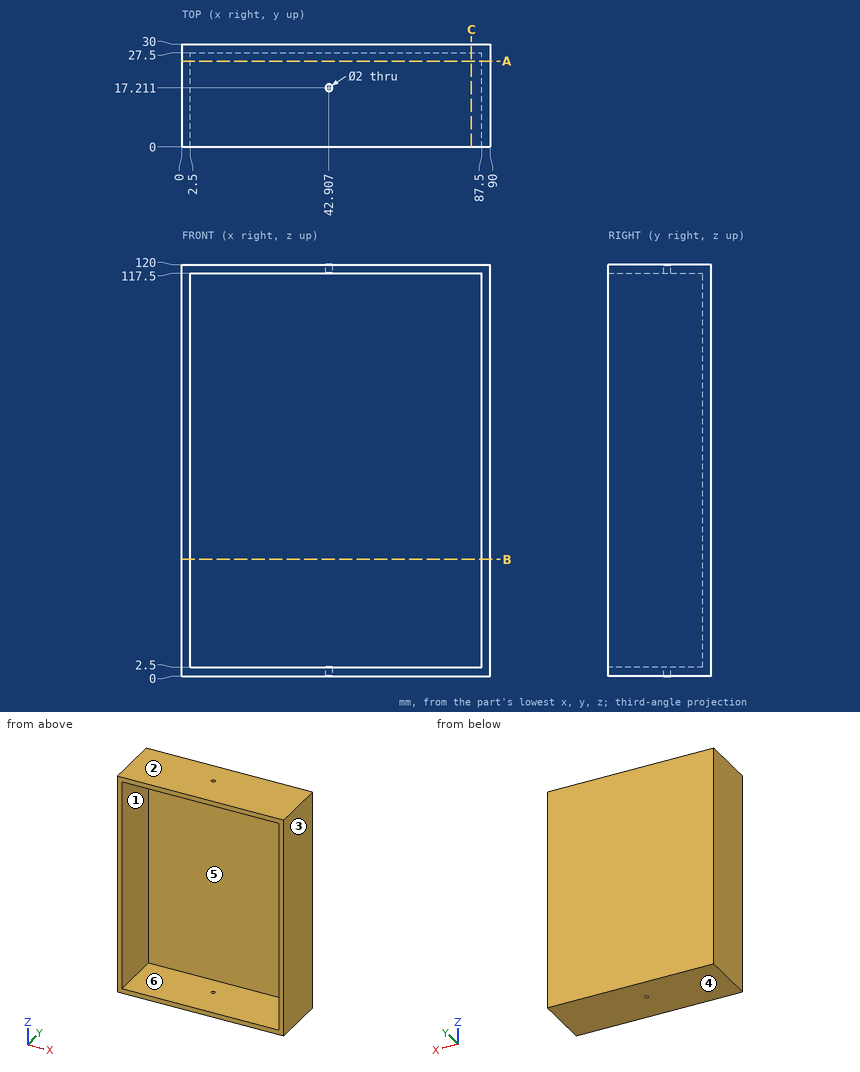
Design review of the part shown in the three views and the two pictorial views. Dimensions are in mm from the part's minimum x, y and z. A direction names the side the tool comes from. Give positions to 0.01 mm unless a question says otherwise; leave off trailing zeros. Loops run counter-clockwise (first coordinate to the right, second up) from the corner with the lowest first, then second, coordinate; pieces in that order, holes last. Notation, with made-up numbers: (-27.75, 64) -> (-10.75, 64) arc R23 ccw to (-10.75, 100) -> close; hole circle Ø4 at (13, 16). An arc over 180 degrees is marked (long way). Put each result on its own line as item: value. Start each with the question number.
1. We need section A-A on y = 25. State the section outline as (x, z) points.
2. For the marked faces 1 and 2, list the 3-axis set-ups (+Z, -Z, +X, -X, +Y, -Y) from which the entire face can be reached by the end or side of a thin tool; tool diameter is ignored.
3. We need section C-C on x = 84.5. State the section outline as (y, z) points.
4. We need section B-B on z = 34. State the section outline as (x, y) points.
5. Wall thickness on probe 1 along Z at (x, y) = (85.5, 5.25); probe 2 along X at (y, z) = (17.25, 66); probe 3 along Y at (x, z) = (21.5, 103): over which ranges is each line inside the solid? List them lowest first.
6. Clearance check with flat-ended pins moving along their axes: P1, Ø1, axis at y = 15.5, z = 95.5, coming from the -X side; P2, Ø4, axis at x = 20, z = 74, coming from the -Y side; P3, Ø1.8, axis at x = 42.91, y = 17.21, coming from the +Z side. State where each tip first meets the part, or that it passes through.
7. Mouldability with a two-part tool opening along Z and no side actions: class the marked faces 3, 4, 5 and 6 as released by +Z, released by -Z, zero draft, split by the parting line, or undercut.
Determined:
1. outline: (0, 0) -> (90, 0) -> (90, 120) -> (0, 120) -> close; hole (2.5, 2.5) -> (87.5, 2.5) -> (87.5, 117.5) -> (2.5, 117.5) -> close
2. face 1: -Y
2. face 2: +Z, +X, -X, +Y, -Y
3. outline: (0, 0) -> (30, 0) -> (30, 120) -> (0, 120) -> (0, 117.5) -> (27.5, 117.5) -> (27.5, 2.5) -> (0, 2.5) -> close
4. outline: (0, 0) -> (2.5, 0) -> (2.5, 27.5) -> (87.5, 27.5) -> (87.5, 0) -> (90, 0) -> (90, 30) -> (0, 30) -> close
5. probe 1: 0 to 2.5, 117.5 to 120
5. probe 2: 0 to 2.5, 87.5 to 90
5. probe 3: 27.5 to 30
6. P1: x = 0
6. P2: y = 27.5
6. P3: through
7. face 3: zero draft
7. face 4: released by -Z
7. face 5: undercut
7. face 6: undercut
